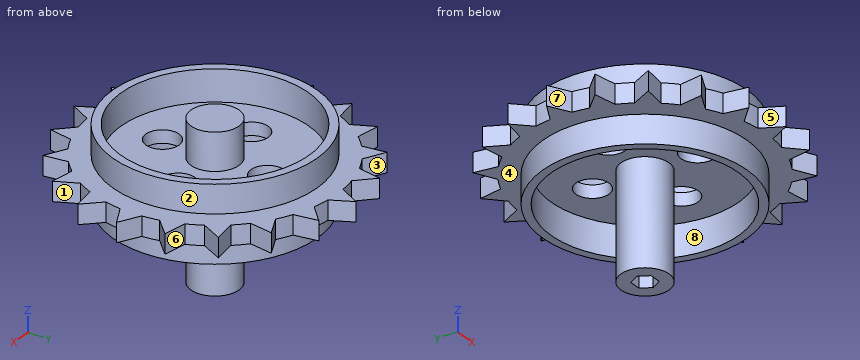
```python
from build123d import *

# Parameters (mm, degrees)
CUT_EXTRUDE2_DEPTH  = 17.78
SKETCH4_R           = 2.189434211
CUT_EXTRUDE3_DEPTH  = 1.6764
BOSS_EXTRUDE1_DEPTH = 2.54


with BuildPart() as part:
    # Sketch1 → Revolve1 (revolve)
    with BuildSketch(Plane(origin=(0, 0, 0), x_dir=(0, 0, -1), z_dir=(1, 0, 0)), mode=Mode.PRIVATE) as revolve1_sk:
        Polygon((4.9657, 13.462), (1.27, 13.462), (1.27, 16.002), (-1.27, 16.002), (-1.27, 13.462), (-4.9657, 13.462), (-4.9657, 12.3698), (-0.8382, 12.3698), (-0.8382, 3.175), (-5.719832453, 3.175), (-5.719832453, 0), (0, 0), (14.625567547, 0), (14.625567547, 3.175), (0.8382, 3.175), (0.8382, 12.3698), (4.9657, 12.3698), align=None)
    revolve(revolve1_sk.sketch.rotate(Axis((0, 0, 0), (0, 0, -1)), 90), axis=Axis((0, 0, 0), (0, 0, -1)))

    # Sketch3 → Cut-Extrude2 (cut)
    with BuildSketch(Plane(origin=(0, 0, -14.625567547), x_dir=(-1, 0, 0), z_dir=(0, 0, -1))):
        Polygon((1.539793168, 0), (0.769896584, 1.3335), (-0.769896584, 1.3335), (-1.539793168, 0), (-0.769896584, -1.3335), (0.769896584, -1.3335), align=None)
    extrude(amount=-CUT_EXTRUDE2_DEPTH, mode=Mode.SUBTRACT)

    # Sketch4 → Cut-Extrude3 (cut)
    with BuildSketch(Plane(origin=(0, 0, -0.8382), x_dir=(-1, 0, 0), z_dir=(0, 0, -1))):
        with Locations((0, 6.954565789)):
            Circle(SKETCH4_R)
        with Locations((6.954565789, 0)):
            Circle(SKETCH4_R)
        with Locations((0, -6.954565789)):
            Circle(SKETCH4_R)
        with Locations((-6.954565789, 0)):
            Circle(SKETCH4_R)
    extrude(amount=-CUT_EXTRUDE3_DEPTH, mode=Mode.SUBTRACT)

    # Sketch5 → Boss-Extrude1 (add)
    with BuildSketch(Plane.XY.offset(1.27)):
        with BuildLine():
            ThreePointArc((-13.73725383, 8.206817971), (-12.945889944, 9.405739607), (-12.050192599, 10.528858548))
            Line((-12.050192599, 10.528858548), (-15.10552331, 10.974805092))
            Line((-15.10552331, 10.974805092), (-13.73725383, 8.206817971))
        make_face()
        with BuildLine():
            ThreePointArc((-10.528858548, 12.050192599), (-9.405739607, 12.945889944), (-8.206817971, 13.73725383))
            Line((-8.206817971, 13.73725383), (-10.974805092, 15.10552331))
            Line((-10.974805092, 15.10552331), (-10.528858548, 12.050192599))
        make_face()
        with BuildLine():
            ThreePointArc((-6.289825233, 14.714010417), (-4.944889944, 15.218806374), (-3.56010282, 15.600950994))
            Line((-3.56010282, 15.600950994), (-5.769796486, 17.757607659))
            Line((-5.769796486, 17.757607659), (-6.289825233, 14.714010417))
        make_face()
        with BuildLine():
            ThreePointArc((-1.4351, 15.937518376), (0, 16.002), (1.4351, 15.937518376))
            Line((1.4351, 15.937518376), (0, 18.671453646))
            Line((0, 18.671453646), (-1.4351, 15.937518376))
        make_face()
        with BuildLine():
            ThreePointArc((3.56010282, 15.600950994), (4.944889944, 15.218806374), (6.289825233, 14.714010417))
            Line((6.289825233, 14.714010417), (5.769796486, 17.757607659))
            Line((5.769796486, 17.757607659), (3.56010282, 15.600950994))
        make_face()
        with BuildLine():
            ThreePointArc((8.206817971, 13.73725383), (9.405739607, 12.945889944), (10.528858548, 12.050192599))
            Line((10.528858548, 12.050192599), (10.974805092, 15.10552331))
            Line((10.974805092, 15.10552331), (8.206817971, 13.73725383))
        make_face()
        with BuildLine():
            ThreePointArc((12.050192599, 10.528858548), (12.945889944, 9.405739607), (13.73725383, 8.206817971))
            Line((13.73725383, 8.206817971), (15.10552331, 10.974805092))
            Line((15.10552331, 10.974805092), (12.050192599, 10.528858548))
        make_face()
        with BuildLine():
            ThreePointArc((14.714010417, 6.289825233), (15.218806374, 4.944889944), (15.600950994, 3.56010282))
            Line((15.600950994, 3.56010282), (17.757607659, 5.769796486))
            Line((17.757607659, 5.769796486), (14.714010417, 6.289825233))
        make_face()
        with BuildLine():
            Line((18.671453646, 0), (16.002, 0))
            ThreePointArc((16.002, 0), (15.985871466, -0.718273954), (15.937518376, -1.4351))
            Line((15.937518376, -1.4351), (18.671453646, 0))
        make_face()
        with BuildLine():
            ThreePointArc((15.937518376, 1.4351), (15.985871466, 0.718273954), (16.002, 0))
            Line((16.002, 0), (18.671453646, 0))
            Line((18.671453646, 0), (15.937518376, 1.4351))
        make_face()
        with BuildLine():
            Line((17.757607659, -5.769796486), (15.600950994, -3.56010282))
            ThreePointArc((15.600950994, -3.56010282), (15.218806374, -4.944889944), (14.714010417, -6.289825233))
            Line((14.714010417, -6.289825233), (17.757607659, -5.769796486))
        make_face()
        with BuildLine():
            Line((15.10552331, -10.974805092), (13.73725383, -8.206817971))
            ThreePointArc((13.73725383, -8.206817971), (12.945889944, -9.405739607), (12.050192599, -10.528858548))
            Line((12.050192599, -10.528858548), (15.10552331, -10.974805092))
        make_face()
        with BuildLine():
            Line((10.974805092, -15.10552331), (10.528858548, -12.050192599))
            ThreePointArc((10.528858548, -12.050192599), (9.405739607, -12.945889944), (8.206817971, -13.73725383))
            Line((8.206817971, -13.73725383), (10.974805092, -15.10552331))
        make_face()
        with BuildLine():
            Line((5.769796486, -17.757607659), (6.289825233, -14.714010417))
            ThreePointArc((6.289825233, -14.714010417), (4.944889944, -15.218806374), (3.56010282, -15.600950994))
            Line((3.56010282, -15.600950994), (5.769796486, -17.757607659))
        make_face()
        with BuildLine():
            Line((0, -18.671453646), (1.4351, -15.937518376))
            ThreePointArc((1.4351, -15.937518376), (0, -16.002), (-1.4351, -15.937518376))
            Line((-1.4351, -15.937518376), (0, -18.671453646))
        make_face()
        with BuildLine():
            Line((-5.769796486, -17.757607659), (-3.56010282, -15.600950994))
            ThreePointArc((-3.56010282, -15.600950994), (-4.944889944, -15.218806374), (-6.289825233, -14.714010417))
            Line((-6.289825233, -14.714010417), (-5.769796486, -17.757607659))
        make_face()
        with BuildLine():
            Line((-10.974805092, -15.10552331), (-8.206817971, -13.73725383))
            ThreePointArc((-8.206817971, -13.73725383), (-9.405739607, -12.945889944), (-10.528858548, -12.050192599))
            Line((-10.528858548, -12.050192599), (-10.974805092, -15.10552331))
        make_face()
        with BuildLine():
            Line((-15.10552331, -10.974805092), (-12.050192599, -10.528858548))
            ThreePointArc((-12.050192599, -10.528858548), (-12.945889944, -9.405739607), (-13.73725383, -8.206817971))
            Line((-13.73725383, -8.206817971), (-15.10552331, -10.974805092))
        make_face()
        with BuildLine():
            Line((-17.757607659, -5.769796486), (-14.714010417, -6.289825233))
            ThreePointArc((-14.714010417, -6.289825233), (-15.218806374, -4.944889944), (-15.600950994, -3.56010282))
            Line((-15.600950994, -3.56010282), (-17.757607659, -5.769796486))
        make_face()
        with BuildLine():
            ThreePointArc((-15.937518376, -1.4351), (-16.002, 0), (-15.937518376, 1.4351))
            Line((-15.937518376, 1.4351), (-18.671453646, 0))
            Line((-18.671453646, 0), (-15.937518376, -1.4351))
        make_face()
        with BuildLine():
            ThreePointArc((-15.600950994, 3.56010282), (-15.218806374, 4.944889944), (-14.714010417, 6.289825233))
            Line((-14.714010417, 6.289825233), (-17.757607659, 5.769796486))
            Line((-17.757607659, 5.769796486), (-15.600950994, 3.56010282))
        make_face()
    extrude(amount=-BOSS_EXTRUDE1_DEPTH)


solid = part.part
```
Here's how the part is built. I have some questions about the finished solid (model axes, mm). Face numbers are marked on the shaded views. A direction names the side the tool comes from. Coordinates: 2 decimals unless noted, no trailing zeros. Order: outer loops, then holes, each group sorted by start corner. A loop starts at its lowest first (then second) coordinate and runs counter-clockwise, first axis right, second up.
Item 1: Which directions (+Z, -Z, +X, -X, +Y, -Y) give clear straight access to the entire face, cutting with the end or side of a thin tool? Please do the marked faces 1, 2, 3, 4 and 5.
Response values:
face 1: +Z, -Z, +X
face 2: +Z
face 3: +Z, -Z, +Y
face 4: -Z
face 5: +Z, -Z, -Y
Item 2: If we section it at A-A, the plane z = -2: Give the number of separate pieces and of enclosed holes in the cut face, then the cut area to 3 significant figures.
Response values:
separate pieces: 2
enclosed holes: 2
area: 114 mm2
Item 3: I'm going to push flat-ended pins straight in: pin 1 Ø4 at (y, z) = (4.5, -4.5) entering from +X; pin 2 Ø11 at (x, y) = (-7.5, -4.5) entering from +Z; pin 3 Ø4 at (y, z) = (6.5, -6) entering from -X. Where does each tip first touch, or does it pass through?
Response values:
pin 1: stops at x = 13.23
pin 2: stops at z = 4.97
pin 3: stops at x = -12.58
Item 4: I need wall thicknesses on probe 1 along Y at (x, z) = (0, -1.7) (1 decimal); probe 2 along Z at (x, y) = (-16, 6); probe 3 along Z at (x, y) = (12, -2). Which ranges of each line are inside material? Lowest first, please.
Response values:
probe 1: y = -13.5 to -12.4, -3.2 to -1.3, 1.3 to 3.2, 12.4 to 13.5
probe 2: z = -1.27 to 1.27
probe 3: z = -0.84 to 0.84
Item 5: If we section it at C-C, the plane x = 7: List the corners of the cut face in (y, z) for me, then the cut area to 3 significant figures.
Response values:
outline: (-14.39, -1.27) - (-11.5, -1.27) - (-11.5, -4.97) - (-10.2, -4.97) - (-10.2, -0.84) - (-2.19, -0.84) - (-2.19, 0.84) - (-10.2, 0.84) - (-10.2, 4.97) - (-11.5, 4.97) - (-11.5, 1.27) - (-14.39, 1.27) - close; (2.19, -0.84) - (10.2, -0.84) - (10.2, -4.97) - (11.5, -4.97) - (11.5, -1.27) - (14.39, -1.27) - (14.39, 1.27) - (11.5, 1.27) - (11.5, 4.97) - (10.2, 4.97) - (10.2, 0.84) - (2.19, 0.84) - close
area: 67.4 mm2
Item 6: Thinking about a two-plate mould opening in X: for the marked faces 6, 7 and 8, which applies, pulls with the +X half, pulls with the -X half, needs draft (parallel to the pull), parting line crosses it, or undercut?
Response values:
face 6: pulls with the +X half
face 7: pulls with the -X half
face 8: undercut
